from build123d import *

# Parameters (mm, degrees)
BOSS_EXTRUDE1_DEPTH = 2.5
CHAMFER1_SIZE       = 0.5


with BuildPart() as part:
    # Sketch1 → Boss-Extrude1 (new body)
    with BuildSketch(Plane(origin=(0, 0, 0), x_dir=(1, 0, 0), z_dir=(0, 1, 0))):
        Polygon((1.662768775, 2.75), (3.250482016, 0), (1.662768775, -2.75), (-1.567505981, -2.75), (-1.567505981, -2.95), (5.682494019, -2.95), (5.682494019, 2.95), (-1.567505981, 2.95), (-1.567505981, 2.75), align=None)
        Polygon((5.682494019, 5), (5.682494019, 2.95), (5.682494019, -2.95), (5.682494019, -5), (8.682494019, -5), (8.682494019, 5), align=None)
    extrude(amount=BOSS_EXTRUDE1_DEPTH)

    # Chamfer1
    chamfer1_edges = [part.edges().sort_by_distance(p)[0] for p in [
        (5.682494019, 1.25, -5),
        (8.682494019, 1.25, -5),
        (8.682494019, 1.25, 5),
        (5.682494019, 1.25, 5),
    ]]
    chamfer(chamfer1_edges, length=CHAMFER1_SIZE)


solid = part.part
Build history of the part. All positions in model axes, mm. A direction names the side the tool comes from. Coordinates: 2 decimals unless noted, no trailing zeros. Order: outer loops, then holes, each group sorted by start corner. A loop starts at its lowest first (then second) coordinate and runs counter-clockwise, first axis right, second up. Notation, with made-up numbers: (-32, 65) - (12, 65) arc R6 ccw to (12, 73) - close; hole circle Ø7 at (49.25, -6.75). An arc over 180 degrees is marked (long way). Write each question's results on one line, items separated by ' | '. Start each with the question number.
Item 1: Wall check: probe 1 along Z at (x, y) = (0.5, 2.2); probe 2 along Z at (x, y) = (5, 0.55); probe 3 along X at (y, z) = (1.75, -3.25). Give the ranges that are in metal, low to high. Write a range as [from, to].
Item 2: Flat gauge pins, fed straight in: pin 1 (2 mm diameter, centred on x = 0.5, z = 1, fed in from +Y); pin 2 (1.2 mm diameter, centred on x = 0.5, y = 1.5, fed in from +Z); pin 3 (1.2 mm diameter, centred on x = 0, y = 1, fed in from -Z); pin 4 (0.5 mm diameter, centred on y = 1, z = -3.5, fed in from -X). Where does each tip first touch, or does it go through?
Item 3: Band-saw the part on C-C on z = 3.75. Write the cut outline in (x, y), and give its area (3 significant figures).
Item 4: Band-saw the part on B-B on y = 0.25. Write the cut outline in (x, z), and give its area (3 significant figures).
Item 5: Band-saw the part on A-A on x = -0.5. Write the cut outline in (y, z).
Item 6: Mould opens along Z. For faces 6 (the face through (2.45, 1.23, -1.39)), 7 (the face through (7, 1, -5)), 8 (the face through (7, 1, 5)) say: released by +Z, released by -Z, zero draft, split by the parting line, or undercut.
Item 7: Tool access for faces 1 (the face through (0, 1, 2.75)), 2 (the face through (6, 0, 0)), 3 (the face through (8.682, 1, 0)), 4 (the face through (2, 1, 2.95)), 5 (the face through (5.682, 1, -4)): list every direction of +Z, -Z, +X, -X, +Y, -Y with a clear straight run to the whole face (end or side of a thin tool).
Item 8: Band-saw the part on D-D on z = 1.25. Write the cut outline in (x, y).
Numbers:
1) probe 1: [-2.95, -2.75], [2.75, 2.95] | probe 2: [-2.95, 2.95] | probe 3: [5.68, 8.68]
2) pin 1: through | pin 2: z = 2.95 | pin 3: z = -2.95 | pin 4: x = 5.68
3) outline: (5.68, 0) - (8.68, 0) - (8.68, 2.5) - (5.68, 2.5) - close | area: 7.50 mm^2
4) outline: (-1.57, -2.95) - (5.68, -2.95) - (5.68, -4.5) - (6.18, -5) - (8.18, -5) - (8.68, -4.5) - (8.68, 4.5) - (8.18, 5) - (6.18, 5) - (5.68, 4.5) - (5.68, 2.95) - (-1.57, 2.95) - (-1.57, 2.75) - (1.66, 2.75) - (3.25, 0) - (1.66, -2.75) - (-1.57, -2.75) - close | area: 50.1 mm^2
5) outline: (0, -2.95) - (2.5, -2.95) - (2.5, -2.75) - (0, -2.75) - close; (0, 2.75) - (2.5, 2.75) - (2.5, 2.95) - (0, 2.95) - close
6) face 6: undercut | face 7: released by -Z | face 8: released by +Z
7) face 1: -X, +Y, -Y | face 2: +Z, -Z, +X, -X, -Y | face 3: +Z, -Z, +X, +Y, -Y | face 4: +Z, -X, +Y, -Y | face 5: -Z, -X, +Y, -Y
8) outline: (2.53, 0) - (8.68, 0) - (8.68, 2.5) - (2.53, 2.5) - close
